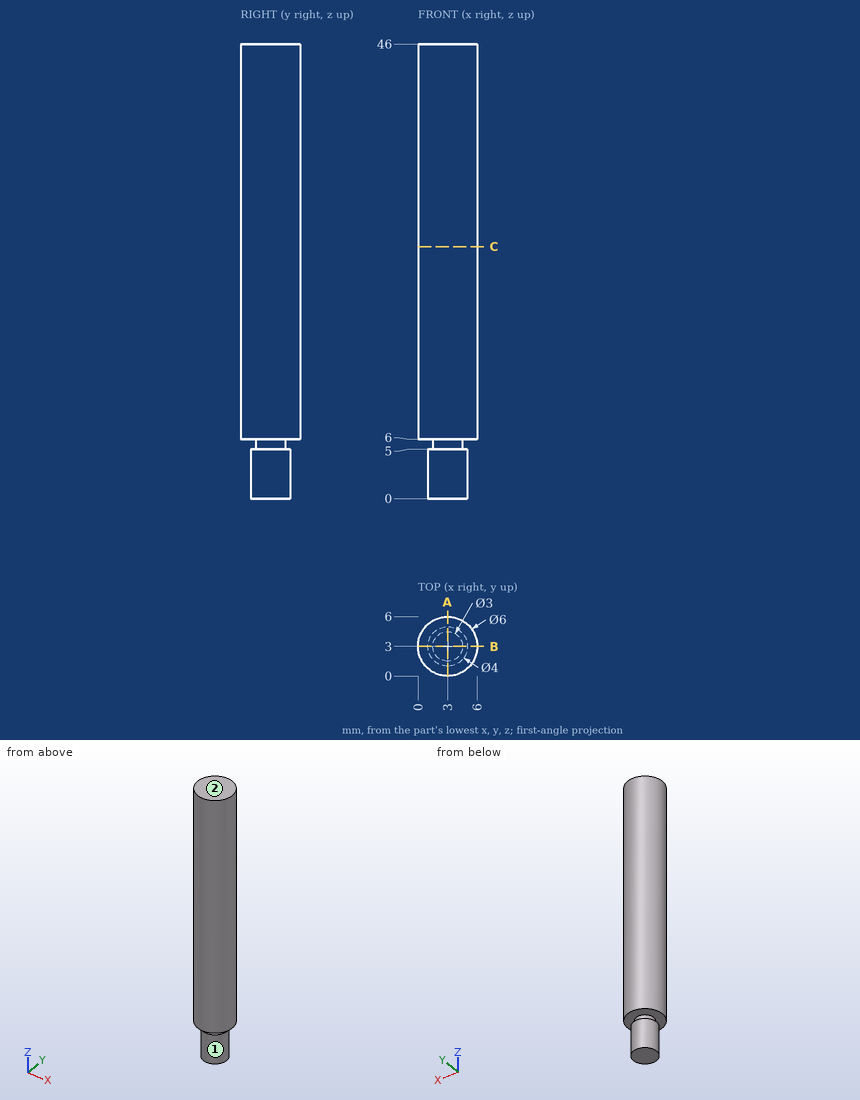
Study the drawing (mm; zero at the part's minimum x, y, z) and answer. A direction names the side the tool comes from. Give positions to 0.01 mm unless a question says otherwise; leave off trailing zeros. Write each loop counter-clockwise with the first axis right and the second up, starting at its lowest first coordinate (ties: lowest second). Pieces come first, ordered by that corner, then holes. Notation, with made-up numbers: (-23, 68) - (17, 68) arc R13 cw to (17, 82) - close; hole circle Ø4 at (22, -36.75). An arc over 180 degrees is marked (long way). Use a Markdown table: item, result.
1. Find the intervals of material crossed by probe 1 along Z at (x, y) = (4.25, 4.5); probe 2 along Y at (x, z) = (2.85, 31); probe 3 along Z at (x, y) = (4.3, 1.35), in increasing order. Write a range as from..to.
Values follow:
| item | result |
|---|---|
| probe 1 | z = 0..5, 6..46 |
| probe 2 | y = 0..6 |
| probe 3 | z = 6..46 |
2. A tool of negligible diameter and unlimited length cuts with its end or side. For the marked faces 1 and 2, from which of +Z, -Z, +X, -X, +Y, -Y can it reach the whole face along a straight path? Write none if from no direction.
Values follow:
| item | result |
|---|---|
| face 1 | -Z |
| face 2 | +Z, +X, -X, +Y, -Y |
3. Section A-A on x = 3 is taken. Write down the section's boundary in (y, z).
Values follow:
| item | result |
|---|---|
| outline | (0, 6) - (1.5, 6) - (1.5, 5) - (1, 5) - (1, 0) - (5, 0) - (5, 5) - (4.5, 5) - (4.5, 6) - (6, 6) - (6, 46) - (0, 46) - close |
4. Each of these flat-tipped pins is pushed along its axis until it touches: P1, Ø1, axis at x = 2, z = 16, coming from the -Y side; P2, Ø1, axis at x = 4.5, z = 31.5, coming from the +Y side. Where does it stop, or does it pass through?
Values follow:
| item | result |
|---|---|
| P1 | stops at y = 0.04 |
| P2 | stops at y = 5.83 |
5. Section C-C on z = 25.5 is taken. Write down the section's boundary in (x, y).
Values follow:
| item | result |
|---|---|
| outline | circle Ø6 at (3, 3) |
